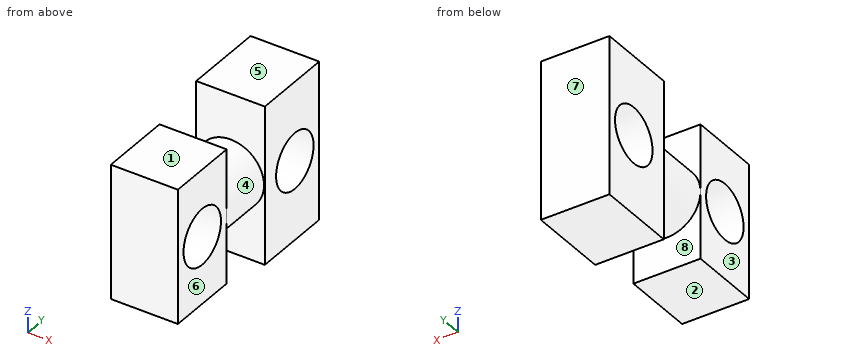
```python
from build123d import *

# Parameters (mm, degrees)
SKETCH1_W           = 12.28
SKETCH1_H           = 14.5
BOSS_EXTRUDE1_DEPTH = 28.28
SKETCH2_R           = 5
CUT_EXTRUDE1_DEPTH  = 28.27
SKETCH3_R           = 6
BOSS_EXTRUDE2_DEPTH = 10
SKETCH4_R           = 6
BOSS_EXTRUDE3_DEPTH = 13
SKETCH5_R           = 5
CUT_EXTRUDE2_DEPTH  = 13


with BuildPart() as part:
    # Sketch1 → Boss-Extrude1 (new body)
    with BuildSketch(Plane.XY):
        with Locations((6.14, 27.98627451)):
            Rectangle(SKETCH1_W, SKETCH1_H)
    extrude(amount=BOSS_EXTRUDE1_DEPTH)

    # Sketch2 → Cut-Extrude1 (cut)
    with BuildSketch(Plane(origin=(12.28, 0, 0), x_dir=(0, 0, -1), z_dir=(1, 0, 0))):
        with Locations(Location((-14.14, 28.73627451, 0), (0, 0, 90))):
            Circle(SKETCH2_R)
    extrude(amount=-CUT_EXTRUDE1_DEPTH, mode=Mode.SUBTRACT)

    # Sketch3 → Boss-Extrude2 (add)
    with BuildSketch(Plane.XZ.offset(-20.73627451)):
        with Locations(Location((6.14, 14.14, 0), (0, 0, 270))):
            Circle(SKETCH3_R)
    extrude(amount=BOSS_EXTRUDE2_DEPTH)

    # Sketch4 → Boss-Extrude3 (add)
    # profile 1 of 2: a face of its own
    with BuildSketch(Plane.XZ.offset(-10.73627451)):
        Polygon((0.14, 26.14), (2.09119792, 26.14), (12.143195084, 26.14), (12.143195084, 2.14), (0.14, 2.14), (0.14, 14.14), align=None)
        with Locations(Location((6.14, 14.14, 0), (0, 0, 180))):
            Circle(SKETCH4_R, mode=Mode.SUBTRACT)
    # profile 2 of 2: a face of its own
    with BuildSketch(Plane.XZ.offset(-10.73627451)):
        with Locations(Location((6.14, 14.14, 0), (0, 0, 180))):
            Circle(SKETCH4_R)
    extrude(amount=BOSS_EXTRUDE3_DEPTH)

    # Sketch5 → Cut-Extrude2 (cut)
    with BuildSketch(Plane.ZY.offset(-0.14)):
        with Locations((14.14, 4.23627451)):
            Circle(SKETCH5_R)
    extrude(amount=-CUT_EXTRUDE2_DEPTH, mode=Mode.SUBTRACT)


solid = part.part
```
Geometry check sheet. Reference: the model listing, model coordinates, mm. Face numbers are marked on the shaded views. A direction names the side the tool comes from. Round coordinates to 2 decimals unless told otherwise and drop trailing zeros. Loops run counter-clockwise (first coordinate to the right, second up) from the corner with the lowest first, then second, coordinate; pieces in that order, holes last. Notation, with made-up numbers: (-21, 20) - (21, 20) arc R26 cw to (21, 49) - close; hole circle Ø3 at (21.25, -23). An arc over 180 degrees is marked (long way). Write item = value, one per line. Start each with the question number.
1. Section check B-B on x = 10.5. Enter the section's corners in (y, z), then the cut area to 3 significant figures.
2. Section check D-D on x = 2. Enter the section's corners in (y, z), then the cut area to 3 significant figures.
3. Mould release check, pull along Y, two halves, no side actions. Record for the marked faces 6, 7 and 8: released by +Y, released by -Y, zero draft, split by the parting line, or undercut.
4. Section check C-C on y = 11.5. Enter the section's corners in (x, z).
5. Set-up check for the marked faces 1, 2, 3, 4 and 5: record each of +Z, -Z, +X, -X, +Y, -Y from which the full face is reachable in a straight line by a thin tool's end or side.
6. Thickness scan on line 1 (Y direction, x = 7, z = 4); line 2 (Z direction, x = 6.5, y = 4.5); line 3 (Y direction, x = 10.75, z = 12). Record the ranges inside material, lowest first.
7. Section check A-A on y = 33. Enter the section's corners in (x, z).
8. Depth check by flat-ended pin: pin 1 (1 mm diameter, centred on x = 2, y = 7.5, fed in from -Z); pin 2 (16 mm diameter, centred on y = 4.24, z = 14.14, fed in from +X). Enter the tip coordinate at first touch or a pass-through.
Working result:
q1.outline = (-2.26, 2.14) - (10.74, 2.14) - (10.74, 10.02) - (20.74, 10.02) - (20.74, 0) - (35.24, 0) - (35.24, 28.28) - (20.74, 28.28) - (20.74, 18.26) - (10.74, 18.26) - (10.74, 26.14) - (-2.26, 26.14) - close; hole circle Ø10 at (4.24, 14.14); hole circle Ø10 at (28.74, 14.14)
q1.area = 647 mm^2
q2.outline = (-2.26, 2.14) - (10.74, 2.14) - (10.74, 9.8) - (20.74, 9.8) - (20.74, 0) - (35.24, 0) - (35.24, 28.28) - (20.74, 28.28) - (20.74, 18.48) - (10.74, 18.48) - (10.74, 26.14) - (-2.26, 26.14) - close; hole circle Ø10 at (4.24, 14.14); hole circle Ø10 at (28.74, 14.14)
q2.area = 652 mm^2
q3.face_6 = zero draft
q3.face_7 = released by +Y
q3.face_8 = undercut
q4.outline = circle Ø12 at (6.14, 14.14)
q5.face_1 = +Z, +X, -X, -Y
q5.face_2 = -Z, +X, -X, -Y
q5.face_3 = +Z, -Z, -X, -Y
q5.face_4 = none
q5.face_5 = +Z, +X, -X, +Y, -Y
q6.line_1 = -2.26 to 10.74, 20.74 to 35.24
q6.line_2 = 2.14 to 9.15, 19.13 to 26.14
q6.line_3 = -2.26 to -0.28, 8.76 to 24.22, 33.26 to 35.24
q7.outline = (0, 0) - (12.28, 0) - (12.28, 11.53) - (0, 11.53) - close; (0, 16.75) - (12.28, 16.75) - (12.28, 28.28) - (0, 28.28) - close
q8.pin_1 = 2.14
q8.pin_2 = 12.14
